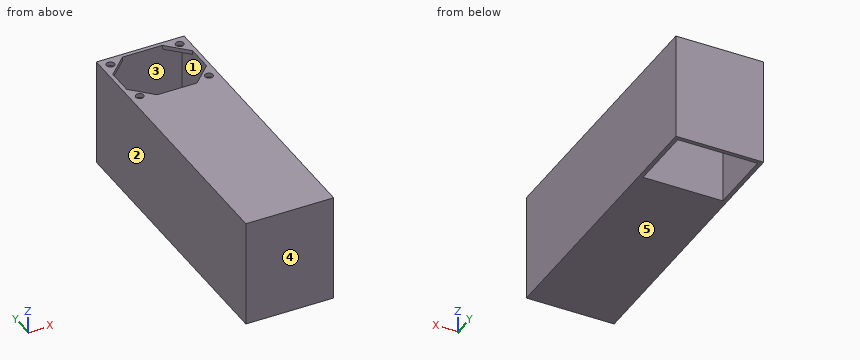
```python
from build123d import *

# Parameters (mm, degrees)
STRUCTURESKETCH_W      = 66
STRUCTURESKETCH_H      = 215
MAINSTRUCTURE_DEPTH    = 81
OBJ1           = 3
CENTERPOCKET_DEPTH     = 81
OBJ2       = 60
OBJ3       = 50
OBJ4 = 78


with BuildPart() as part:
    # StructureSketch → MainStructure (new body)
    with BuildSketch(Plane.XY):
        Rectangle(STRUCTURESKETCH_W, STRUCTURESKETCH_H)
    extrude(amount=MAINSTRUCTURE_DEPTH)

    with BuildSketch(Plane(origin=(0, 79.5, 0), x_dir=(1, 0, 0), z_dir=(0, 0, 1))):
        with Locations((-26, 21)):
            Circle(OBJ1)
        with Locations((26, 21)):
            Circle(OBJ1)
        with Locations((26, -21)):
            Circle(OBJ1)
        with Locations((-26, -21)):
            Circle(OBJ1)
        Polygon((-15, 25), (15, 25), (30, 10), (30, -10), (15, -25), (-15, -25), (-30, -10), (-30, 10), align=None)
    extrude(amount=CENTERPOCKET_DEPTH, mode=Mode.SUBTRACT)

    with BuildSketch(Plane(origin=(0, 79.5, 0), x_dir=(1, 0, 0), z_dir=(0, 0, 1))):
        Rectangle(OBJ2, OBJ3)
    extrude(amount=OBJ4, mode=Mode.SUBTRACT)


solid = part.part
```
The model under review builds one solid part; all positions refer to its coordinate system, in mm. Face numbers are marked on the shaded views. A direction names the side the tool comes from. Round coordinates to 2 decimals unless told otherwise and drop trailing zeros. Loops run counter-clockwise (first coordinate to the right, second up) from the corner with the lowest first, then second, coordinate; pieces in that order, holes last. Notation, with made-up numbers: (-12, 27) -> (0, 27) arc R9 cw to (0, 40) -> close; hole circle Ø6 at (38.5, 74). An arc over 180 degrees is marked (long way). Answer as a JSON object with one key per item and string values. Group by question number.
1) We need section B-B on x = -1.5. Write out the cut boundary in (y, z).
2) For the marked faces 1 and 2, list the 3-axis set-ups (+Z, -Z, +X, -X, +Y, -Y) from which the entire face can be reached by the end or side of a thin tool; tool diameter is ignored.
3) We need section D-D on y = 87. Write out the cut boundary in (x, z).
4) For line 1 (Y direction, x = 23, z = 48.5); line 2 (Y direction, x = 26, z = 79.3); line 3 (X direction, y = 100.5, z = 80.3), list the stretches that pass through material, from the lowest coordinate up. Write a range as [from, to].
5) For pin 1 Ø4.5 at (x, y) = (20.5, 94) entering from -Z; pin 2 Ø7.5 at (x, y) = (25, 59) entering from -Z, all flat-tipped, find the tip position at first contact; note any pin that passes through.
6) We need section A-A on y = 58.5. Write out the cut boundary in (x, z), then the cut area to 3 significant figures.
7) Mouldability with a two-part tool opening along Y and no side actions: class the marked faces 3, 4 and 5 as released by +Y, released by -Y, zero draft, split by the parting line, or undercut.
8) We need section C-C on x = -26. Write out the cut boundary in (y, z), then the cut area to 3 significant figures.
Result set:
{
 "1": {"outline": "(-107.5, 0) -> (54.5, 0) -> (54.5, 81) -> (-107.5, 81) -> close; (104.5, 0) -> (107.5, 0) -> (107.5, 81) -> (104.5, 81) -> close"},
 "2": {"face 1": "-Z", "face 2": "+Z, -Z, -X, +Y, -Y"},
 "3": {"outline": "(-33, 0) -> (-30, 0) -> (-30, 81) -> (-33, 81) -> close; (30, 0) -> (33, 0) -> (33, 81) -> (30, 81) -> close"},
 "4": {"line 1": "[-107.5, 54.5], [104.5, 107.5]", "line 2": "[-107.5, 55.5], [61.5, 65.5], [93.5, 97.5], [103.5, 107.5]", "line 3": "[-33, -29], [-23, -19], [19, 23], [29, 33]"},
 "5": {"pin 1": "through", "pin 2": "z = 78"},
 "6": {"outline": "(-33, 0) -> (-30, 0) -> (-30, 78) -> (-29, 78) -> (-29, 81) -> (-33, 81) -> close; (-23, 78) -> (-19, 78) -> (-19, 81) -> (-23, 81) -> close; (19, 78) -> (23, 78) -> (23, 81) -> (19, 81) -> close; (29, 78) -> (30, 78) -> (30, 0) -> (33, 0) -> (33, 81) -> (29, 81) -> close", "area": "516 mm²"},
 "7": {"face 3": "undercut", "face 4": "released by -Y", "face 5": "zero draft"},
 "8": {"outline": "(-107.5, 0) -> (54.5, 0) -> (54.5, 78) -> (55.5, 78) -> (55.5, 81) -> (-107.5, 81) -> close; (61.5, 78) -> (65.5, 78) -> (65.5, 81) -> (61.5, 81) -> close; (93.5, 78) -> (97.5, 78) -> (97.5, 81) -> (93.5, 81) -> close; (103.5, 78) -> (104.5, 78) -> (104.5, 0) -> (107.5, 0) -> (107.5, 81) -> (103.5, 81) -> close", "area": "13,400 mm²"}
}
